Work out the finished part from the listing and answer in its coordinate system (mm). A direction names the side the tool comes from. Round coordinates to 2 decimals unless told otherwise and drop trailing zeros. Write each loop counter-clockwise with the first axis right and the second up, starting at its lowest first coordinate (ties: lowest second). Pieces come first, ordered by that corner, then holes.
1. Find section A-A (y = 0). Write down the section's boundary in (x, z), and give its area (3 significant figures).
2. Flat-ended cylindrical pins translate along their axes: pin 1 Ø1 at (x, y) = (-0.5, 0.5) entering from +Z; pin 2 Ø1 at (x, y) = (11, 1) entering from -Z; pin 3 Ø1.5 at (y, z) = (1, 0.5) entering from +X. Find the tip coordinate at first contact, or state that the pin passes through.
3. A tool of negligible diameter and unlimited length cuts with its end or side. For faces 1 (the face through (0.1, 1.03, 0.79)), 2 (the face through (-20, 0, 0)), from which of +Z, -Z, +X, -X, +Y, -Y can it reach the whole face along a straight path? Write none if from no direction.
4. Find section D-D (x = 14.5). Write down the section's boundary in (y, z).
5. Find section C-C (x = 3.5). Write down the section's boundary in (y, z).
6. Straight lines are drawn through the part: probe 1 along Z at (x, y) = (-17.5, -0.1); probe 2 along Z at (x, y) = (13, 1.1); probe 3 along Y at (x, z) = (11, -0.6). For each, find the intervals that lie inside material, in ascending order.
```python
from build123d import *


with BuildPart() as part:
    # 草图1 → Revolve 558 (revolve)
    with BuildSketch(Plane.XY, mode=Mode.PRIVATE) as revolve_558_sk:
        Polygon((-20, 1.5), (-8, 1.5), (-7.25, 1.299), (7.25, 1.299), (8, 1.5), (20, 1.5), (20, 0), (-20, 0), align=None)
    revolve(revolve_558_sk.sketch.rotate(Axis((-20, 0, 0), (1, 0, 0)), 180), axis=Axis((-20, 0, 0), (1, 0, 0)))

    # 草图2 → Cut-Revolve 802 (revolve, cut)
    with BuildSketch(Plane.XY, mode=Mode.PRIVATE) as cut_revolve_802_sk:
        Polygon((-20.249992667, 1.5), (-19.750007333, 1.5), (-20, 1.067), align=None)
    cut_revolve_802 = revolve(cut_revolve_802_sk.sketch.rotate(Axis((-26.952426469, 0, 0), (1, 0, 0)), 180), axis=Axis((-26.952426469, 0, 0), (1, 0, 0)), mode=Mode.SUBTRACT)

    # 镜向1: Cut-Revolve 802 across plane
    add(cut_revolve_802.mirror(Plane(origin=(0, 0, 0), x_dir=(0, 0, 1), z_dir=(1, 0, 0))), mode=Mode.SUBTRACT)


solid = part.part
```
Worked answers:
1. outline: (-20, -1.07) - (-19.75, -1.5) - (-8, -1.5) - (-7.25, -1.3) - (7.25, -1.3) - (8, -1.5) - (19.75, -1.5) - (20, -1.07) - (20, 1.07) - (19.75, 1.5) - (8, 1.5) - (7.25, 1.3) - (-7.25, 1.3) - (-8, 1.5) - (-19.75, 1.5) - (-20, 1.07) - close
1. area: 114 mm2
2. pin 1: stops at z = 1.3
2. pin 2: stops at z = -1.41
2. pin 3: stops at x = 20
3. face 1: none
3. face 2: +Z, -Z, -X, +Y, -Y
4. outline: circle Ø3 at (0, 0)
5. outline: circle Ø2.6 at (0, 0)
6. probe 1: z = -1.5 to 1.5
6. probe 2: z = -1.02 to 1.02
6. probe 3: y = -1.37 to 1.37
